Geometry: final body of the model. Coordinates: model frame, mm. A direction names the side the tool comes from. Coordinates: 2 decimals unless noted, no trailing zeros. Loops run counter-clockwise (first coordinate to the right, second up) from the corner with the lowest first, then second, coordinate; pieces in that order, holes last. Notation, with made-up numbers: (35, 19) - (58, 19) arc R26 cw to (58, 58) - close; hole circle Ø6 at (49, -36). An arc over 180 degrees is marked (long way). Put each result on its own line as item: value. Start each with the question number.
1) Section B-B on y = 30. Output: boundary loops of the cut face in (x, z).
2) Material intervals for line 1 along Y through (x, z) = (37.5, 1.35); line 2 along X through (y, z) = (10.5, 1.55); line 3 along X through (y, z) = (53.5, 1.2), sorted ascending. Write a range as from..to.
3) Draft query along Y for faces 5 (the flat face through (63, 15, 1)), 6 (the flat face through (53.25, 45, 1)), 7 (the flat face through (61.75, 3, 1)). Return one class per face: +Y half, -Y half, draft (parallel to the pull), parting line (faces both ways), or undercut.
4) Section D-D on x = 21. Output: boundary loops of the cut face in (y, z).
5) Contact query for flat-ended pins moving along their axis: pin 1 Ø1.5 at (x, z) = (63.5, 2) entering from -Y; pin 2 Ø0.9 at (x, z) = (34, 2) entering from -Y; pin 3 Ø1.2 at (x, z) = (65.5, 2) entering from +Y; pin 4 Ø0.9 at (y, z) = (62, 1.5) entering from -X. Output: stop coordinate, or through.
6) Section C-C on z = 0.8. Count the separate pieces of the cut face and the enclosed holes in it, and give its area (3 significant figures).
7) Section A-A on y = 20. Output: boundary loops of the cut face in (x, z).
8) Reachability of faces 1 (the flat face through (10, -2, 1)), 2 (the flat face through (56.75, 45, 1)), 3 (the flat face through (32, 60, 1)), 4 (the flat face through (12, 45, 1)) from +Z, -Z, +X, -X, +Y, -Y: full face, straight path, thin tool, end or side. Return the list, or none.
```python
from build123d import *

# Parameters (mm, degrees)
ESQUISSE1_R        = 4.1
ESQUISSE1_R_2      = 1.5
ESQUISSE1_W        = 1.5
ESQUISSE1_H        = 12.1
BOSS_EXTRU_1_DEPTH = 3


with BuildPart() as part:
    # Esquisse1 → Boss.-Extru.1 (new body)
    with BuildSketch(Plane.XY):
        Polygon((0, 0), (10, 0), (10, -5), (25, -5), (25, 0), (61.75, 0), (61.75, 6), (60.25, 6), (60.25, 9), (61.75, 9), (61.75, 15), (65, 15), (65, 9), (66.5, 9), (66.5, 6), (65, 6), (65, 0), (75, 0), (75, 60), (65, 60), (65, 65), (50, 65), (50, 60), (13.25, 60), (13.25, 54), (14.75, 54), (14.75, 51), (13.25, 51), (13.25, 45), (10, 45), (10, 51), (8.5, 51), (8.5, 54), (10, 54), (10, 60), (0, 60), align=None)
        with Locations((37.5, 30)):
            Circle(ESQUISSE1_R, mode=Mode.SUBTRACT)
        with Locations((25, 20)):
            Circle(ESQUISSE1_R_2, mode=Mode.SUBTRACT)
        with Locations(Location((50, 20, 0), (0, 0, 180))):
            Circle(ESQUISSE1_R_2, mode=Mode.SUBTRACT)
        with BuildLine():
            Line((30.75, 38.9), (53.25, 38.9))
            Line((53.25, 38.9), (53.25, 51))
            Line((53.25, 51), (30.75, 51))
            add(Edge.make_bspline(
                [(30.75, 51), (27.25, 51), (27.25, 44.95), (27.25, 38.9), (30.75, 38.9)],
                knots=[3.141592654, 3.141592654, 3.141592654, 4.71238898, 4.71238898, 6.283185307, 6.283185307, 6.283185307], degree=2, weights=[1, 0.707106781, 1, 0.707106781, 1]))
        make_face(mode=Mode.SUBTRACT)
        with Locations((56, 44.95)):
            Rectangle(ESQUISSE1_W, ESQUISSE1_H, mode=Mode.SUBTRACT)
    extrude(amount=BOSS_EXTRU_1_DEPTH)


solid = part.part
```
Answer block:
1. outline: (0, 0) - (33.4, 0) - (33.4, 3) - (0, 3) - close; (41.6, 0) - (75, 0) - (75, 3) - (41.6, 3) - close
2. line 1: y = 0..25.9, 34.1..38.9, 51..60
2. line 2: x = 0..61.75, 65..75
2. line 3: x = 0..8.5, 14.75..75
3. face 5: -Y half
3. face 6: undercut
3. face 7: draft
4. outline: (-5, 0) - (60, 0) - (60, 3) - (-5, 3) - close
5. pin 1: stops at y = 15
5. pin 2: stops at y = 0
5. pin 3: stops at y = 65
5. pin 4: stops at x = 50
6. separate pieces: 1
6. enclosed holes: 5
6. area: 4,140 mm²
7. outline: (0, 0) - (23.5, 0) - (23.5, 3) - (0, 3) - close; (26.5, 0) - (48.5, 0) - (48.5, 3) - (26.5, 3) - close; (51.5, 0) - (75, 0) - (75, 3) - (51.5, 3) - close
8. face 1: +Z, -Z, -X, -Y
8. face 2: +Z, -Z
8. face 3: +Z, -Z, -X, +Y
8. face 4: +Z, -Z, +Y
